from build123d import *

# Parameters (mm, degrees)
F0_R     = 40
F0_R_2   = 35.5
F1_DEPTH = 10
F0_R_3   = 30.5
F0_R_4   = 26


with BuildPart() as f1:
    # F0 (on Top) → F1 (new body)
    with BuildSketch(Plane.XY):
        Circle(F0_R)
        Circle(F0_R_2, mode=Mode.SUBTRACT)
    extrude(amount=F1_DEPTH)


with BuildPart() as f1b:
    # F0 (on Top) → F1, piece 2 (new body)
    with BuildSketch(Plane.XY):
        Circle(F0_R_3)
        Circle(F0_R_4, mode=Mode.SUBTRACT)
    extrude(amount=F1_DEPTH)


solid = f1b.part
Geometry check sheet. Reference: the model listing, model coordinates, mm. Give positions to 0.01 mm unless a question says otherwise; leave off trailing zeros. Write each loop counter-clockwise with the first axis right and the second up, starting at its lowest first coordinate (ties: lowest second). Pieces come first, ordered by that corner, then holes.
1) Go/stop test with flat-tipped pins: pin 1 Ø3 at (x, y) = (23.5, -1.5) entering from +Z; pin 2 Ø2 at (x, z) = (24, 7.5) entering from +Y; pin 3 Ø2 at (x, z) = (4, 4) entering from -Y; pin 4 Ø3 at (x, z) = (-12, 3) entering from +Y. Record where each tip stops, or that it passes through.
Values follow:
pin 1: passes through
pin 2: stops at y = 20.03
pin 3: stops at y = -30.35
pin 4: stops at y = 28.64
2) Cross-section at A-A (y = 0). Record the boundary of the cut face in (x, z).
Values follow:
outline: (-30.5, 0) - (-26, 0) - (-26, 10) - (-30.5, 10) - close; (26, 0) - (30.5, 0) - (30.5, 10) - (26, 10) - close
3) Release check for a two-part mould opening along Y. For faces 1 (the face through (22.5, 13.7, 10)), 2 (the face through (-20.633, -15.821, 4.93)), 3 (the face through (-24.204, -18.559, 4.93)) record: released by +Y, released by -Y, zero draft, split by the parting line, or undercut.
Values follow:
face 1: zero draft
face 2: undercut
face 3: split by the parting line
4) Cross-section at C-C (z = 6.75). Record the boundary of the cut face in (x, y).
Values follow:
outline: circle Ø61 at (0, 0); hole circle Ø52 at (0, 0)
5) Thickness scan on line 1 (Y direction, x = 0, z = 8); line 2 (Y direction, x = -4.5, z = 8); line 3 (X direction, y = 18, z = 7.75). Record the ranges inside material, lowest first.
Values follow:
line 1: y = -30.5 to -26, 26 to 30.5
line 2: y = -30.17 to -25.61, 25.61 to 30.17
line 3: x = -24.62 to -18.76, 18.76 to 24.62
